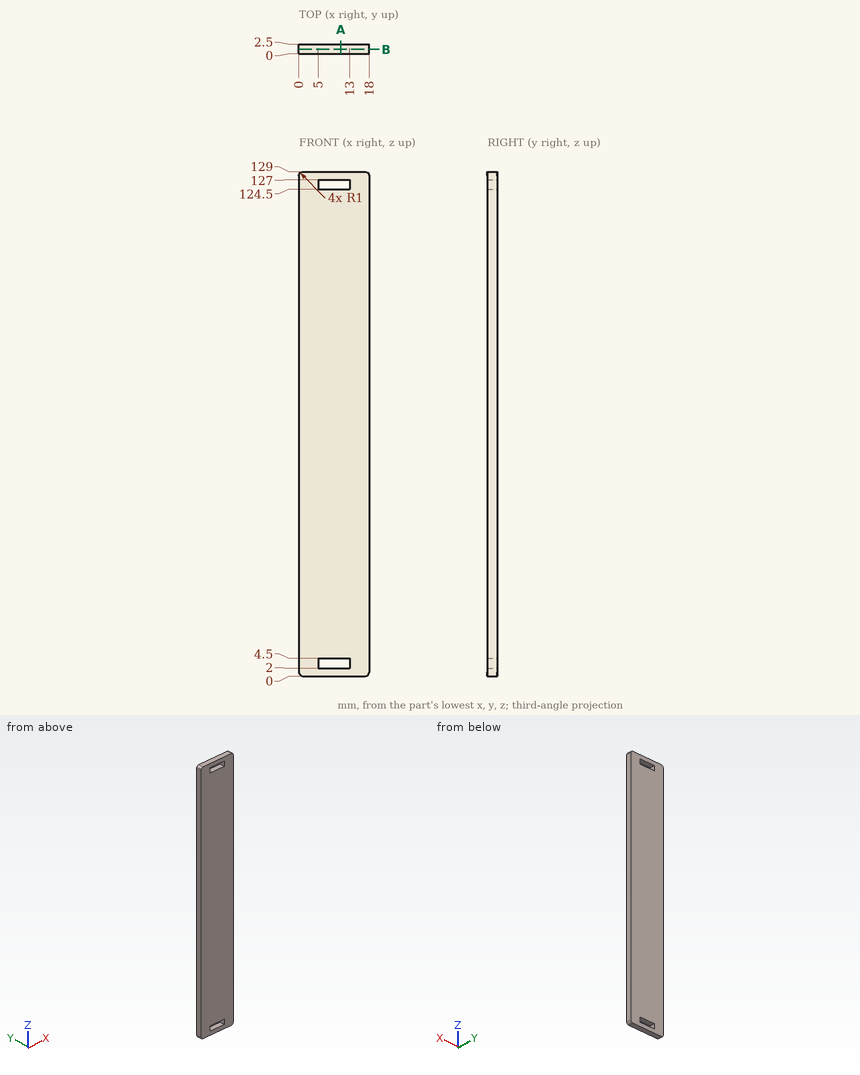
Check sheet for the drawn part. Datum: minimum x, y, z corner. Units: mm. Coordinates: 2 decimals unless noted, no trailing zeros. Order: outer loops, then holes, each group sorted by start corner. A loop starts at its lowest first (then second) coordinate and runs counter-clockwise, first axis right, second up. Notation, with made-up numbers: (53.25, -20) -> (103.25, -20) arc R15 cw to (103.25, 0) -> close; hole circle Ø5 at (-30, 44). An arc over 180 degrees is marked (long way). Use a Markdown table: item, result. Add a question column.
1. Cross-section at B-B (y = 1.15). Enter the section's corners in (x, z).
2. Cross-section at A-A (x = 10.75). Enter the section's corners in (y, z), and give its area (3 significant figures).
3. Go/stop test with a flat-tipped pin: pin 1 Ø2 at (x, z) = (3, 104.5) entering from -Y. Record where the tip stops, or that it passes through.
4. Material ranges on L1, parallel to Z at x = 5.25, y = 1.95, recorded low to high.
Filled sheet:
| question | item | result |
|---|---|---|
| 1 | outline | (0, 1) arc R1 ccw to (1, 0) -> (17, 0) arc R1 ccw to (18, 1) -> (18, 128) arc R1 ccw to (17, 129) -> (1, 129) arc R1 ccw to (0, 128) -> close; hole (5, 2) -> (13, 2) -> (13, 4.5) -> (5, 4.5) -> close; hole (5, 124.5) -> (13, 124.5) -> (13, 127) -> (5, 127) -> close |
| 2 | outline | (0, 0) -> (2.5, 0) -> (2.5, 2) -> (0, 2) -> close; (0, 4.5) -> (2.5, 4.5) -> (2.5, 124.5) -> (0, 124.5) -> close; (0, 127) -> (2.5, 127) -> (2.5, 129) -> (0, 129) -> close |
| 2 | area | 310 mm2 |
| 3 | pin 1 | y = 0 |
| 4 | L1 | 0 to 2, 4.5 to 124.5, 127 to 129 |
